Source: CAD feature listing. Evaluate the final solid. Frame: model axes, mm. Face numbers are marked on the shaded views. A direction names the side the tool comes from. Give positions to 0.01 mm unless a question says otherwise; leave off trailing zeros. Loops run counter-clockwise (first coordinate to the right, second up) from the corner with the lowest first, then second, coordinate; pieces in that order, holes last.
from build123d import *

# Parameters (mm, degrees)
F0_W      = 101.6
F0_H      = 76.2
F1_DEPTH  = 25.4
F2_R      = 31.75
F3_DEPTH  = 25.4
F3_FACE_R = 31.75
F4_DEPTH  = 50.801
F5_R      = 5.884043
F6_DEPTH  = 25.401
F7_R      = 7.500717
F8_DEPTH  = 25.401
F10_DEPTH = 19.05
F12_DEPTH = 19.05
F14_DEPTH = 19.05
F16_DEPTH = 19.05
F18_DEPTH = 25.4


with BuildPart() as f1:
    # F0 (on Front) → F1 (new body)
    with BuildSketch(Plane.XZ):
        with Locations((50.8, 38.1)):
            Rectangle(F0_W, F0_H)
    extrude(amount=F1_DEPTH)

    # F2 (on face) → F3 (join)
    with BuildSketch(Plane.XZ.offset(25.4)):
        with Locations((50.8, 38.1)):
            Circle(F2_R)
    extrude(amount=F3_DEPTH)

    # F3_face (on face) → F4 (cut, through all)
    with BuildSketch(Plane(origin=(50.8, -50.8, 38.1), x_dir=(1, 0, 0), z_dir=(0, -1, 0))):
        Circle(F3_FACE_R)
    extrude(amount=-F4_DEPTH, mode=Mode.SUBTRACT)

    # F5 (on face) → F6 (cut, through all)
    with BuildSketch(Plane.XZ.offset(25.4)):
        with Locations((8.164548, 68.496935)):
            Circle(F5_R)
    extrude(amount=-F6_DEPTH, mode=Mode.SUBTRACT)

    # F7 (on face) → F8 (cut, through all)
    with BuildSketch(Plane.XZ.offset(25.4)):
        with Locations((85.848674, 66.40365)):
            Circle(F7_R)
    extrude(amount=-F8_DEPTH, mode=Mode.SUBTRACT)

    # F9 (on face) → F10 (cut)
    with BuildSketch(Plane.XY.offset(76.2)):
        Polygon((73.521554, -3.837689), (52.356116, -3.837689), (63.75289, -15.46705), align=None)
    extrude(amount=-F10_DEPTH, mode=Mode.SUBTRACT)

    # F11 (on face) → F12 (cut)
    with BuildSketch(Plane.XY.offset(76.2)):
        Polygon((26.538938, -3.372515), (7.931962, -3.372515), (8.397136, -6.861323), (22.119781, -6.861323), (22.119781, -22.444667), (26.538938, -22.444667), (40.49417, -22.444667), (40.49417, -15.234463), (26.538938, -15.234463), align=None)
    extrude(amount=-F12_DEPTH, mode=Mode.SUBTRACT)

    # F13 (on face) → F14 (cut)
    with BuildSketch(Plane.XY.offset(76.2)):
        Polygon((98.640978, -5.465799), (81.662104, -5.465799), (68.172053, -21.049144), (98.640978, -21.049144), align=None)
    extrude(amount=-F14_DEPTH, mode=Mode.SUBTRACT)

    # F15 (on face) → F16 (cut)
    with BuildSketch(Plane(origin=(0, 0, 0), x_dir=(1, 0, 0), z_dir=(0, 0, -1))):
        Polygon((18.863561, 23.375014), (3.280218, 23.375014), (3.280218, 19.188445), (13.746641, 19.188445), (13.746641, 8.489433), (18.398385, 8.489433), (31.888444, 8.489433), (31.888444, 2.209579), (69.567569, 2.209579), (69.567569, 5.698387), (86.546443, 5.698387), (86.546443, 10.582718), (86.546443, 16.629985), (96.547693, 16.629985), (96.547693, 21.746906), (83.290212, 21.746906), (83.290212, 11.280479), (64.915828, 11.280479), (64.915828, 3.605102), (36.772776, 3.605102), (36.772776, 11.280479), (18.863561, 11.280479), align=None)
    extrude(amount=-F16_DEPTH, mode=Mode.SUBTRACT)

    # F17 (on face) → F18 (join)
    with BuildSketch(Plane.YZ.offset(101.6)):
        Polygon((-23.375014, 28.724518), (-11.978242, 18.955858), (-15.001875, 8.72202), (-6.861323, 18.955858), (-2.209579, 24.537953), (-6.861323, 28.414406), (-1.256352, 35.140372), (-6.861323, 36.632486), (-13.606353, 48.959609), (-13.606353, 36.632486), align=None)
    extrude(amount=F18_DEPTH)


solid = f1.part
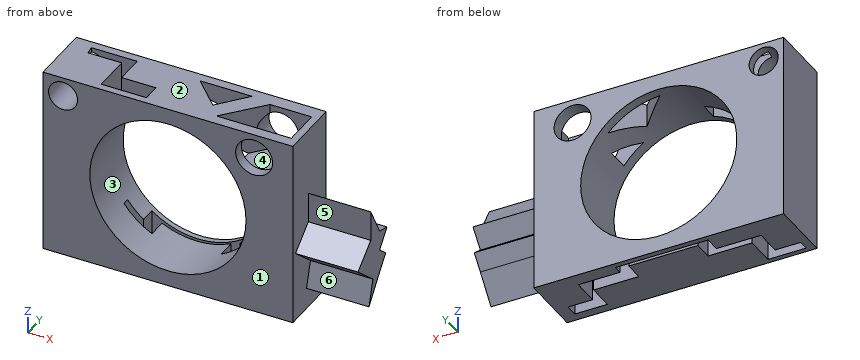
1) Reachability of the marked faces 4, 5 and 6 from +Z, -Z, +X, -X, +Y, -Y: full face, straight path, thin tool, end or side. Return the list, or none.
Checks:
face 4: +Z
face 5: +Z, +X, -Y
face 6: +X, -Y
2) Ray query, probe 1 along Y at (x, z) = (18.5, 61); probe 2 along Y at (x, z) = (23.5, 17); probe 3 along X at (y, z) = (-4.5, 11). Return the intervals inside material, ascending.
Checks:
probe 1: y = -25.4 to -6.86, -3.37 to 0
probe 2: y = -25.4 to -11.28, -8.49 to 0
probe 3: x = 0 to 31.89, 69.57 to 101.6
3) Cut plane A-A (x = 50.8). Return loops of the section in (y, z), and give its area (3 significant figures).
Checks:
outline: (-25.4, 0) - (-3.61, 0) - (-3.61, 6.35) - (-25.4, 6.35) - close; (-25.4, 69.85) - (0, 69.85) - (0, 76.2) - (-25.4, 76.2) - close; (-2.21, 0) - (0, 0) - (0, 6.35) - (-2.21, 6.35) - close
area: 314 mm2
4) Contact query for flat-ended pins moving along their axis: P1, Ø3, axis at y = -12.5, z = 8.5, coming from the +X side; P2, Ø3, axis at x = 110, y = -7, coming from the -Z side. Output: stop coordinate, or through.
Checks:
P1: stops at x = 101.6
P2: stops at z = 16.9
5) Cut plane D-D (x = 35.5). Return loops of the section in (y, z).
Checks:
outline: (-25.4, 0) - (-11.28, 0) - (-11.28, 10.28) - (-25.4, 10.28) - close; (-25.4, 65.92) - (-22.44, 65.92) - (-22.44, 76.2) - (-25.4, 76.2) - close; (-15.23, 65.92) - (0, 65.92) - (0, 76.2) - (-15.23, 76.2) - close; (-2.21, 0) - (0, 0) - (0, 10.28) - (-2.21, 10.28) - close
6) Cut plane C-C (x = 17). Return loops of the section in (y, z), and give its area (3 significant figures).
Checks:
outline: (-25.4, 0) - (-23.38, 0) - (-23.38, 19.05) - (-8.49, 19.05) - (-8.49, 0) - (0, 0) - (0, 76.2) - (-3.37, 76.2) - (-3.37, 57.15) - (-6.86, 57.15) - (-6.86, 76.2) - (-25.4, 76.2) - close
area: 1,590 mm2
7) Pull-direction query (Z, two-part tool) for the marked faces 1, 2 and 3; classes: released by +Z, released by -Z, zero draft, split by the parting line, or undercut.
Checks:
face 1: zero draft
face 2: released by +Z
face 3: undercut
8) Cut plane B-B (z = 38.1). Return loops of the section in (x, y), and give its area (3 significant figures).
Checks:
outline: (0, -25.4) - (19.05, -25.4) - (19.05, 0) - (0, 0) - close; (82.55, -25.4) - (101.6, -25.4) - (101.6, -13.61) - (127, -13.61) - (127, -7.66) - (101.6, -7.66) - (101.6, 0) - (82.55, 0) - close
area: 1,120 mm2
